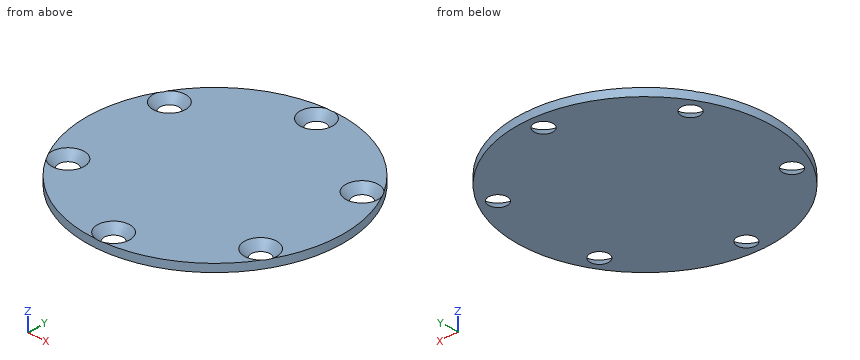
```python
from build123d import *

# Parameters (mm, degrees)
SKETCH1_R                                     = 25.4
BOSS_EXTRUDE1_DEPTH                           = 1.5875
CSK_FOR_4_FLAT_HEAD_SOCKET_CAP_SCREW1_A_COUNT = 2
CSK_FOR_4_FLAT_HEAD_SOCKET_CAP_SCREW1_A_PITCH = 22.225
CSK_FOR_4_FLAT_HEAD_SOCKET_CAP_SCRE_2_COUNT   = 2
CSK_FOR_4_FLAT_HEAD_SOCKET_CAP_SCRE_2_PITCH   = 38.494829198
CSK_FOR_4_FLAT_HEAD_SOCKET_CAP_SCRE_3_COUNT   = 2
CSK_FOR_4_FLAT_HEAD_SOCKET_CAP_SCRE_3_PITCH   = 44.45
CSK_FOR_4_FLAT_HEAD_SOCKET_CAP_SCRE_4_COUNT   = 2
CSK_FOR_4_FLAT_HEAD_SOCKET_CAP_SCRE_4_PITCH   = 38.494829198
CSK_FOR_4_FLAT_HEAD_SOCKET_CAP_SCRE_5_COUNT   = 2
CSK_FOR_4_FLAT_HEAD_SOCKET_CAP_SCRE_5_PITCH   = 22.225


with BuildPart() as part:
    # Sketch1 → Boss-Extrude1 (new body)
    with BuildSketch(Plane.XY):
        Circle(SKETCH1_R)
    extrude(amount=BOSS_EXTRUDE1_DEPTH)

    # Sketch3 → CSK for #4 Flat Head Socket Cap Screw1 (revolve, cut)
    with BuildSketch(Plane(origin=(0, 22.225, 1.5875), x_dir=(0, -1, 0), z_dir=(1, 0, 0))):
        Polygon((0, 0), (0, 1.5875), (1.63195, 1.5875), (1.63195, 1.848124365), (3.2385, 0), align=None)
    csk_for_4_flat_head_socket_cap_screw1 = revolve(axis=Axis((0, 22.225, 7.9375), (0, 0, -1)), mode=Mode.SUBTRACT)

    # CSK for #4 Flat Head Socket Cap Screw1 a: CSK for #4 Flat Head Socket Cap Screw1 ×2
    with Locations(*[Vector(0.866025403784438, -0.500000000000001, 0) * (i * CSK_FOR_4_FLAT_HEAD_SOCKET_CAP_SCREW1_A_PITCH) for i in range(1, CSK_FOR_4_FLAT_HEAD_SOCKET_CAP_SCREW1_A_COUNT)]):
        add(csk_for_4_flat_head_socket_cap_screw1, mode=Mode.SUBTRACT)

    # CSK for _4 Flat Head Socket Cap Scre 2: CSK for #4 Flat Head Socket Cap Screw1 ×2
    with Locations(*[Vector(0.5000000000000123, -0.8660254037844316, 0) * (i * CSK_FOR_4_FLAT_HEAD_SOCKET_CAP_SCRE_2_PITCH) for i in range(1, CSK_FOR_4_FLAT_HEAD_SOCKET_CAP_SCRE_2_COUNT)]):
        add(csk_for_4_flat_head_socket_cap_screw1, mode=Mode.SUBTRACT)

    # CSK for _4 Flat Head Socket Cap Scre 3: CSK for #4 Flat Head Socket Cap Screw1 ×2
    with Locations(*[(0, -i * CSK_FOR_4_FLAT_HEAD_SOCKET_CAP_SCRE_3_PITCH, 0) for i in range(1, CSK_FOR_4_FLAT_HEAD_SOCKET_CAP_SCRE_3_COUNT)]):
        add(csk_for_4_flat_head_socket_cap_screw1, mode=Mode.SUBTRACT)

    # CSK for _4 Flat Head Socket Cap Scre 4: CSK for #4 Flat Head Socket Cap Screw1 ×2
    with Locations(*[Vector(-0.4999999999999876, -0.8660254037844458, 0) * (i * CSK_FOR_4_FLAT_HEAD_SOCKET_CAP_SCRE_4_PITCH) for i in range(1, CSK_FOR_4_FLAT_HEAD_SOCKET_CAP_SCRE_4_COUNT)]):
        add(csk_for_4_flat_head_socket_cap_screw1, mode=Mode.SUBTRACT)

    # CSK for _4 Flat Head Socket Cap Scre 5: CSK for #4 Flat Head Socket Cap Screw1 ×2
    with Locations(*[Vector(-0.8660254037844416, -0.49999999999999495, 0) * (i * CSK_FOR_4_FLAT_HEAD_SOCKET_CAP_SCRE_5_PITCH) for i in range(1, CSK_FOR_4_FLAT_HEAD_SOCKET_CAP_SCRE_5_COUNT)]):
        add(csk_for_4_flat_head_socket_cap_screw1, mode=Mode.SUBTRACT)


solid = part.part
```
The listing builds one solid part. Answer for the finished solid, in the listing's coordinates (mm). Coordinates: 2 decimals unless noted, no trailing zeros. Loops run counter-clockwise (first coordinate to the right, second up) from the corner with the lowest first, then second, coordinate; pieces in that order, holes last. Notation, with made-up numbers: (86.25, -10.5) -> (122.25, -10.5) arc R17 ccw to (122.25, 0.5) -> close; hole circle Ø8 at (-39, 40.25). An arc over 180 degrees is marked (long way). Use one line per item in the form item = value. Start each with the question number.
Item 1: The part is cut by section A-A on z = 0.9. Determine the outline of the cut face in (x, y) (1 decimal), then the cut area to 3 significant figures.
Item 2: The part is cut by section C-C on y = 7. Determine the outline of the cut face in (x, z), then the cut area to 3 significant figures.
Item 3: The part is cut by section D-D on x = 6.5. Determine the outline of the cut face in (y, z), then the cut area to 3 significant figures.
Item 4: The part is cut by section B-B on x = 0. Determine the outline of the cut face in (y, z).
Item 5: Consider L1, parallel to Y at x = -20, z = 0.65; L2, parallel to X at y = 11, z = 1.5; L3, parallel to X at y = 11.5, z = 1.5. Determine where each line is inside the solid, lowest interval first. Write a range as [from, to].
Answer key:
q1.outline = circle Ø50.8 at (0, 0); hole circle Ø5.3 at (-19.2, -11.1); hole circle Ø5.3 at (-19.2, 11.1); hole circle Ø5.3 at (0, -22.2); hole circle Ø5.3 at (0, 22.2); hole circle Ø5.3 at (19.2, -11.1); hole circle Ø5.3 at (19.2, 11.1)
q1.area = 1,900 mm2
q2.outline = (-24.42, 0) -> (24.42, 0) -> (24.42, 1.59) -> (-24.42, 1.59) -> close
q2.area = 77.5 mm2
q3.outline = (-24.55, 0) -> (24.55, 0) -> (24.55, 1.59) -> (-24.55, 1.59) -> close
q3.area = 78.0 mm2
q4.outline = (-25.4, 0) -> (-24.08, 0) -> (-25.4, 1.51) -> close; (-20.37, 0) -> (20.37, 0) -> (18.99, 1.59) -> (-18.99, 1.59) -> close; (24.08, 0) -> (25.4, 0) -> (25.4, 1.51) -> close
q5.L1 = [-15.66, -13.42], [-8.81, 8.81], [13.42, 15.66]
q5.L2 = [-22.89, -22.41], [-16.09, 16.09], [22.41, 22.89]
q5.L3 = [-22.65, -22.39], [-16.11, 16.11], [22.39, 22.65]
